Job drawing, mm, ordinate dimensions from the low corner. One solid piece. Round coordinates to 2 decimals unless told otherwise and drop trailing zeros. Loops run counter-clockwise (first coordinate to the right, second up) from the corner with the lowest first, then second, coordinate; pieces in that order, holes last.
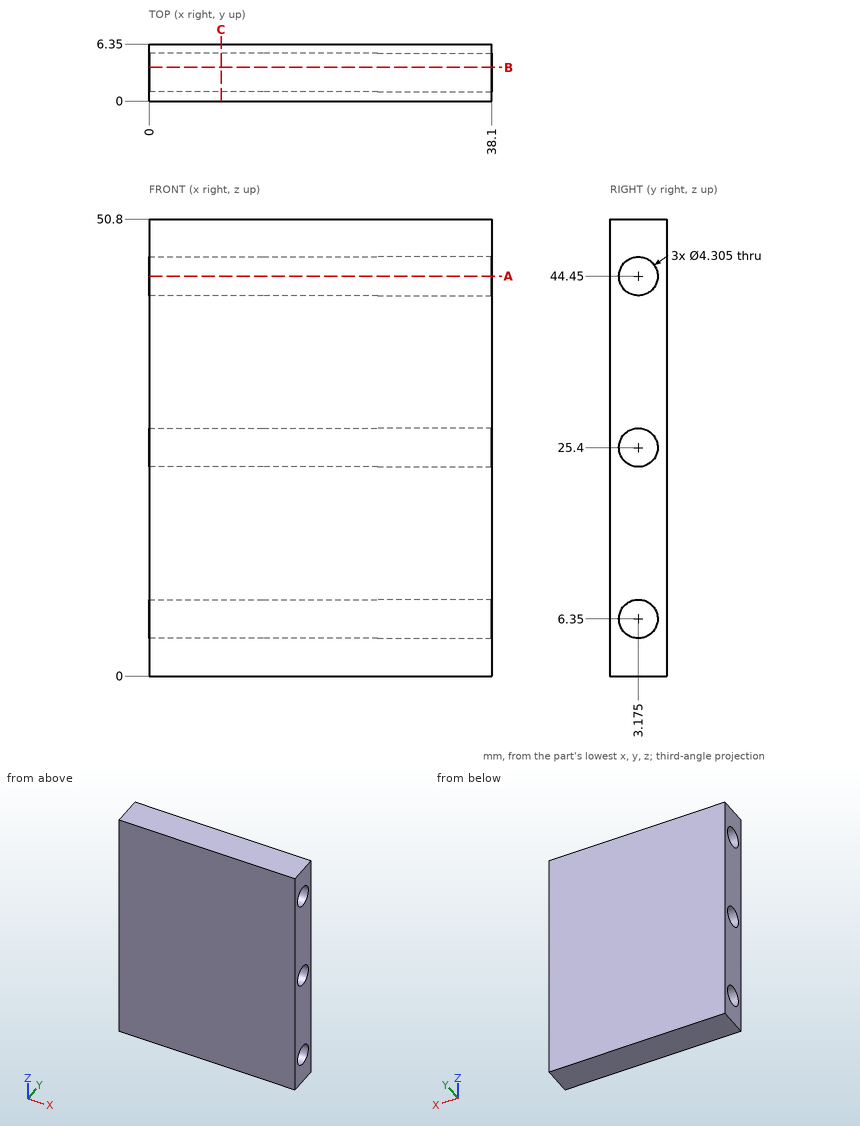
1) Slice it at C-C, the plane x = 8. Give the number of separate pieces and of enclosed holes in the cut face, then the cut area to 3 significant figures.
Values:
separate pieces: 1
enclosed holes: 3
area: 279 mm2
2) Slice it at B-B, the plane y = 3.75. Give the cut face in (x, z) (1 decimal), then the cut area to 3 significant figures.
Values:
outline: (0, 0) - (38.1, 0) - (38.1, 4.3) - (0, 4.3) - close; (0, 8.4) - (38.1, 8.4) - (38.1, 23.3) - (0, 23.3) - close; (0, 27.5) - (38.1, 27.5) - (38.1, 42.4) - (0, 42.4) - close; (0, 46.5) - (38.1, 46.5) - (38.1, 50.8) - (0, 50.8) - close
area: 1,460 mm2
3) Slice it at A-A, the plane z = 44.45. Give the cut face in (x, y).
Values:
outline: (0, 0) - (38.1, 0) - (38.1, 1.02) - (0, 1.02) - close; (0, 5.33) - (38.1, 5.33) - (38.1, 6.35) - (0, 6.35) - close
4) Wall check: line 1 along Z through (x, y) = (33, 3) (1 decimal); line 2 along Z through (x, y) = (7.5, 2.25); line 3 along Y through (x, z) = (33.5, 44.45). Give the ranges that are in metal, low to high.
Values:
line 1: z = 0 to 4.2, 8.5 to 23.3, 27.5 to 42.3, 46.6 to 50.8
line 2: z = 0 to 4.41, 8.29 to 23.46, 27.34 to 42.51, 46.39 to 50.8
line 3: y = 0 to 1.02, 5.33 to 6.35
5) Drop a flat-ended pin along its axis: pin 1 Ø2.5 at (y, z) = (3.175, 25.4) entering from -X. Give the stop position or say it passes through.
Values:
pin 1: passes through
